Here's how the part is built. I have some questions about the finished solid (model axes, mm). Coordinates: 2 decimals unless noted, no trailing zeros. Write each loop counter-clockwise with the first axis right and the second up, starting at its lowest first coordinate (ties: lowest second). Pieces come first, ordered by that corner, then holes. Notation, with made-up numbers: M -0.75,49.5 L 33.25,49.5 A15 cw 33.25,73.5 Z; hole C 71.25,34 d8. An arc over 180 degrees is marked long. Use one line per item in the form item = value. Start each with the question number.
1. Please list where these lines run through material, in increasing order: line 1 along Y through (x, z) = (17.5, 3.35); line 2 along Y through (x, z) = (-60.5, 1.45). Write a range as [from, to].
2. I want a section at D-D, the plane z = 3.15. List the corners of the cut face in (x, y) for me.
3. I want a section at A-A, the plane x = -15. List the corners of the cut face in (y, z) for me, plus the area to 3 significant figures.
4. I want a section at C-C, the plane y = -65. List the corners of the cut face in (x, z) for me, plus the area to 3 significant figures.
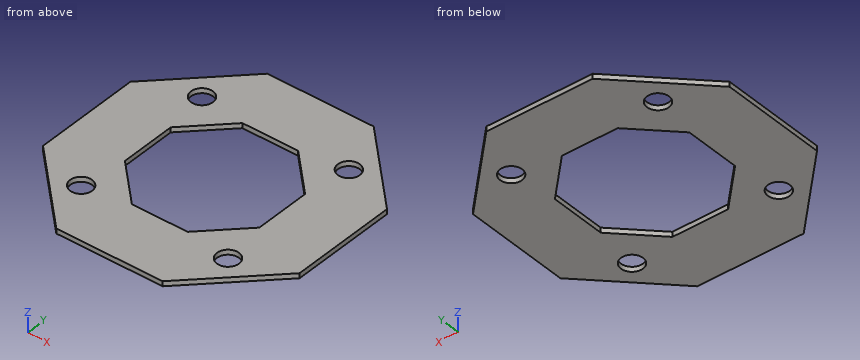
Autodesk Inventor part; units mm, degrees
ref_plane "YZ Plane" through (0, 0, 0) normal (1, 0, 0) x (0, 1, 0)
ref_plane "XZ Plane" through (0, 0, 0) normal (0, 1, 0) x (-1, 0, 0)
ref_plane "XY Plane" through (0, 0, 0) normal (0, 0, 1) x (1, 0, 0)
sketch "Sketch1" plane through (0, 0, 0) normal (0, 0, 1) x (1, 0, 0)
  circle A0 centre (0, 0) radius 55 construction
  circle A1 centre (0, 0) radius 105 construction
  line L0 (105, -105) -> (-105, -105)
  line L1 (-105, -105) -> (-105, 105)
  line L2 (-105, 105) -> (105, 105)
  line L3 (105, 105) -> (105, -105)
  line L4 (105, -105) -> (-105, 105) construction
  line L5 (-105, -105) -> (105, 105) construction
  line L6 (43.4924, 105) -> (105, 43.4924)
  line L7 (105, 43.4924) -> (105, -43.4924)
  line L8 (105, -43.4924) -> (43.4924, -105)
  line L9 (43.4924, -105) -> (-43.4924, -105)
  line L10 (-43.4924, -105) -> (-105, -43.4924)
  line L11 (-105, -43.4924) -> (-105, 43.4924)
  line L12 (-105, 43.4924) -> (-43.4924, 105)
  line L13 (-43.4924, 105) -> (43.4924, 105)
  line L14 (22.7817, 55) -> (55, 22.7817)
  line L15 (55, 22.7817) -> (55, -22.7817)
  line L16 (55, -22.7817) -> (22.7817, -55)
  line L17 (22.7817, -55) -> (-22.7817, -55)
  line L18 (-22.7817, -55) -> (-55, -22.7817)
  line L19 (-55, -22.7817) -> (-55, 22.7817)
  line L20 (-55, 22.7817) -> (-22.7817, 55)
  line L21 (-22.7817, 55) -> (22.7817, 55)
  point P0 (0, 105)
  point P1 (-105, 43.4924)
  point P2 (-43.4924, -105)
  point P3 (0, 55)
  dimension "d22" = 110
  dimension "d23" = 210
extrude "Plate1" add sketch "Sketch1" along normal blind 4 contours L0 L10 L1 L12 L2 L6 L3 L8
sketch "Sketch6" plane through (0, 0, 0) normal (0, 0, 1) x (1, 0, 0)
  line L0 (0, 0) -> (0, 85) construction
  circle A0 centre (0, 0) radius 85 construction
  line L1 (0, 0) -> (60.1041, 60.1041) construction
  circle A1 centre (60.1041, 60.1041) radius 9
  dimension "d32" = 18
  dimension "d33" = 170
  dimension "d34" = 45
extrude "Cut2" cut sketch "Sketch6" along normal blind 4
pattern_circular "Circular Pattern2" count 4 over 360 about axis through (0, 0, -10) along (0, 0, 1) of "Cut2"
equation "\"d23\" = Flange_D_outer"
equation "\"d32\" = Flange_d_hole_diam"
equation "\"d33\" = Flange_D1_hole_center"
equation "\"d35\" = Thickness"
equation "\"d2\" = Thickness"
equation "\"BendReliefWidth\" = Thickness"
equation "\"BendReliefDepth\" = 0.5 * Thickness"
equation "\"CornerReliefSize\" = 4 * Thickness"
equation "\"MinimumRemnant\" = 2 * Thickness"
equation "\"TransitionRadius\" = BendRadius"
equation "\"JacobiRadiusSize\" = BendRadius"
equation "\"GapSize\" = Thickness"
properties part number "DSB 110 drain sustem flange" material "Stainless Steel"
Answer list:
q1.line_1 = [-105, -55], [55, 105]
q1.line_2 = [-87.99, -69.1], [-51.11, 51.11], [69.1, 87.99]
q2.outline = M -105,-43.49 L -43.49,-105 L 43.49,-105 L 105,-43.49 L 105,43.49 L 43.49,105 L -43.49,105 L -105,43.49 Z; hole C -60.1,-60.1 d18; hole C -60.1,60.1 d18; hole M -55,-22.78 L -22.78,-55 L 22.78,-55 L 55,-22.78 L 55,22.78 L 22.78,55 L -22.78,55 L -55,22.78 Z; hole C 60.1,-60.1 d18; hole C 60.1,60.1 d18
q3.outline = M -105,0 L -55,0 L -55,4 L -105,4 Z; M 55,0 L 105,0 L 105,4 L 55,4 Z
q3.area = 400 mm²
q4.outline = M -83.49,0 L -67.66,0 L -67.66,4 L -83.49,4 Z; M -52.55,0 L 52.55,0 L 52.55,4 L -52.55,4 Z; M 67.66,0 L 83.49,0 L 83.49,4 L 67.66,4 Z
q4.area = 547 mm²
